Part model, mm, in its own coordinate system. Face numbers are marked on the shaded views. A direction names the side the tool comes from. Give positions to 0.01 mm unless a question says otherwise; leave off trailing zeros. Order: outer loops, then holes, each group sorted by start corner. A loop starts at its lowest first (then second) coordinate and runs counter-clockwise, first axis right, second up. Notation, with made-up numbers: (60, -33) -> (113, -33) arc R30 cw to (113, 6) -> close; hole circle Ø6 at (-16, 36.25). An arc over 180 degrees is marked (long way). Write item = value, one per line. Start each with the question number.
(1) Probe line 1 along Y through (x, z) = (37, 4.5); line 2 along Z through (x, y) = (11.5, 28). List the from-to ranges inside material, lowest first. Write a range as from..to.
(2) Saw through at A-A, the plane x = 7.5. List the corners of the cut face in (y, z).
(3) Saw through at B-B, the plane z = 11.5. List the corners of the cut face in (x, y).
(4) Saw through at D-D, the plane z = 37. List the corners of the cut face in (x, y).
(5) Which spindle directions (+Z, -Z, +X, -X, +Y, -Y) get a long thin tool onto all of the face, cutting with end or side? Do the marked faces 1 and 2. Say none if no direction does.
(6) Saw through at C-C, the plane x = 32. List the corners of the cut face in (y, z).
(7) Flat gauge pins, fed straight in: pin 1 (3 mm diameter, centred on x = 7.5, y = 40.07, fed in from -Z); pin 2 (10 mm diameter, centred on x = 7, z = 10, fed in from +Y); pin 3 (6 mm diameter, centred on x = 4.5, y = 24, fed in from +Z); pin 4 (25 mm diameter, centred on y = 23.5, z = 37, fed in from +X). Where does each tip first touch, or does it go through?
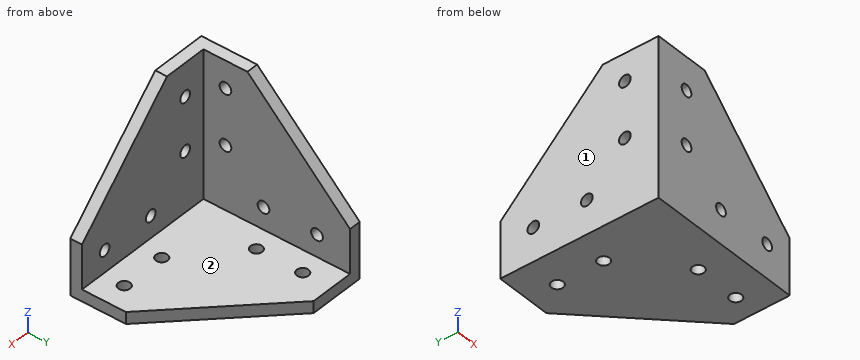
from build123d import *

# Parameters (mm, degrees)
F0_R     = 2
F1_DEPTH = 4
F2_R     = 2
F3_DEPTH = 4
F4_R     = 2
F5_DEPTH = 4


with BuildPart() as f1:
    # F0 (on Top) → F1 (new body)
    with BuildSketch(Plane.XY):
        Polygon((15, 50), (0, 50), (-4, 50), (-4, 0), (-4, -4), (50, -4), (50, 0), (50, 15), align=None)
        with Locations((26.219012, 7.5)):
            Circle(F0_R, mode=Mode.SUBTRACT)
        with Locations((41.652899, 7.5)):
            Circle(F0_R, mode=Mode.SUBTRACT)
        with Locations((7.5, 24.26653)):
            Circle(F0_R, mode=Mode.SUBTRACT)
        with Locations((7.5, 40.072314)):
            Circle(F0_R, mode=Mode.SUBTRACT)
    extrude(amount=F1_DEPTH)

    # F2 (on face) → F3 (join)
    with BuildSketch(Plane.XZ.offset(4)):
        Polygon((-4, 54), (-4, 4), (50, 4), (50, 19), (15, 54), align=None)
        with Locations((21.682408, 11.5)):
            Circle(F2_R, mode=Mode.SUBTRACT)
        with Locations((7.5, 24.480278)):
            Circle(F2_R, mode=Mode.SUBTRACT)
        with Locations((40.694896, 11.5)):
            Circle(F2_R, mode=Mode.SUBTRACT)
        with Locations((7.5, 42.723257)):
            Circle(F2_R, mode=Mode.SUBTRACT)
    extrude(amount=-F3_DEPTH)

    # F4 (on face) → F5 (join)
    with BuildSketch(Plane(origin=(-4, 0, 0), x_dir=(0, -1, 0), z_dir=(-1, 0, 0))):
        Polygon((-50, 0), (0, 0), (0, 54), (-15, 54), (-50, 19), align=None)
        with Locations((-38.723257, 11.5)):
            Circle(F4_R, mode=Mode.SUBTRACT)
        with Locations((-20.480278, 11.5)):
            Circle(F4_R, mode=Mode.SUBTRACT)
        with Locations((-7.5, 25.682408)):
            Circle(F4_R, mode=Mode.SUBTRACT)
        with Locations((-7.5, 44.694896)):
            Circle(F4_R, mode=Mode.SUBTRACT)
    extrude(amount=-F5_DEPTH)


solid = f1.part
Results list:
q1.line_1 = -4..0
q1.line_2 = 0..4
q2.outline = (-4, 0) -> (22.27, 0) -> (22.27, 4) -> (0, 4) -> (0, 22.48) -> (-4, 22.48) -> close; (-4, 26.48) -> (0, 26.48) -> (0, 40.72) -> (-4, 40.72) -> close; (-4, 44.72) -> (0, 44.72) -> (0, 54) -> (-4, 54) -> close; (26.27, 0) -> (38.07, 0) -> (38.07, 4) -> (26.27, 4) -> close; (42.07, 0) -> (50, 0) -> (50, 4) -> (42.07, 4) -> close
q3.outline = (-4, -4) -> (19.68, -4) -> (19.68, 0) -> (0, 0) -> (0, 18.48) -> (-4, 18.48) -> close; (-4, 22.48) -> (0, 22.48) -> (0, 36.72) -> (-4, 36.72) -> close; (-4, 40.72) -> (0, 40.72) -> (0, 50) -> (-4, 50) -> close; (23.68, -4) -> (38.69, -4) -> (38.69, 0) -> (23.68, 0) -> close; (42.69, -4) -> (50, -4) -> (50, 0) -> (42.69, 0) -> close
q4.outline = (-4, -4) -> (32, -4) -> (32, 0) -> (0, 0) -> (0, 32) -> (-4, 32) -> close
q5.face_1 = +Z, -Z, -X, +Y, -Y
q5.face_2 = +Z, +X, +Y
q6.outline = (-4, 0) -> (33, 0) -> (33, 4) -> (0, 4) -> (0, 37) -> (-4, 37) -> close
q7.pin_1 = through
q7.pin_2 = 0
q7.pin_3 = 4
q7.pin_4 = 0
